Can you work these out from the drawing? Everything is in mm from the part's minimum corner. A direction names the side the tool comes from. Round coordinates to 2 decimals unless told otherwise and drop trailing zeros. Write each loop counter-clockwise with the first axis right and the second up, starting at its lowest first coordinate (ties: lowest second). Pieces come first, ordered by that corner, then holes. Notation, with made-up numbers: (-15, 13) -> (26, 13) arc R16 cw to (26, 31) -> close; hole circle Ø11 at (54, 71). An arc over 180 degrees is marked (long way). Answer as CSV lines item,"result". Start each with the question number.
Q1. For the marked faces 5, 6 and 7, which set-ups out of +Z, -Z, +X, -X, +Y, -Y let a thin tool reach every point of the face, with its end or its side?
Q2. If we mould it in two halves opening along X, with no side actions, what happens to the marked faces 1, 2, 3 and 4? For each: pulls with the +X half, pulls with the -X half, needs draft (parallel to the pull), parting line crosses it, or undercut.
Q3. If I drill on line 1 (Z direction, x = 12.7, y = 6.75); line 2 (Y direction, x = 76.5, z = 31) (1 decimal); line 3 (Y direction, x = 115.5, z = 10.5), over which ranges is the centre line in solid material (lowest first)? Write a range as [from, to].
Q4. Will these pins go through, and if not, where does the flat tip stop? pin 1 Ø17.5 at (x, z) = (9, 24.5) entering from +Y; pin 2 Ø4.5 at (x, z) = (12.7, 12.7) entering from -Y; pin 3 Ø1.6 at (y, z) = (14.5, 31.5) entering from -X (3 decimals); pin 4 Ø15 at (x, z) = (50.5, 45) entering from -Y (3 decimals).
Q5. Imagine slicing it at D-D on x = 97.5. Please give me the cut outline in (y, z).
Q6. Imagine slicing it at A-A on y = 1.75. Give the number of separate pieces and of enclosed holes in the cut face, and give its area (3 significant figures).
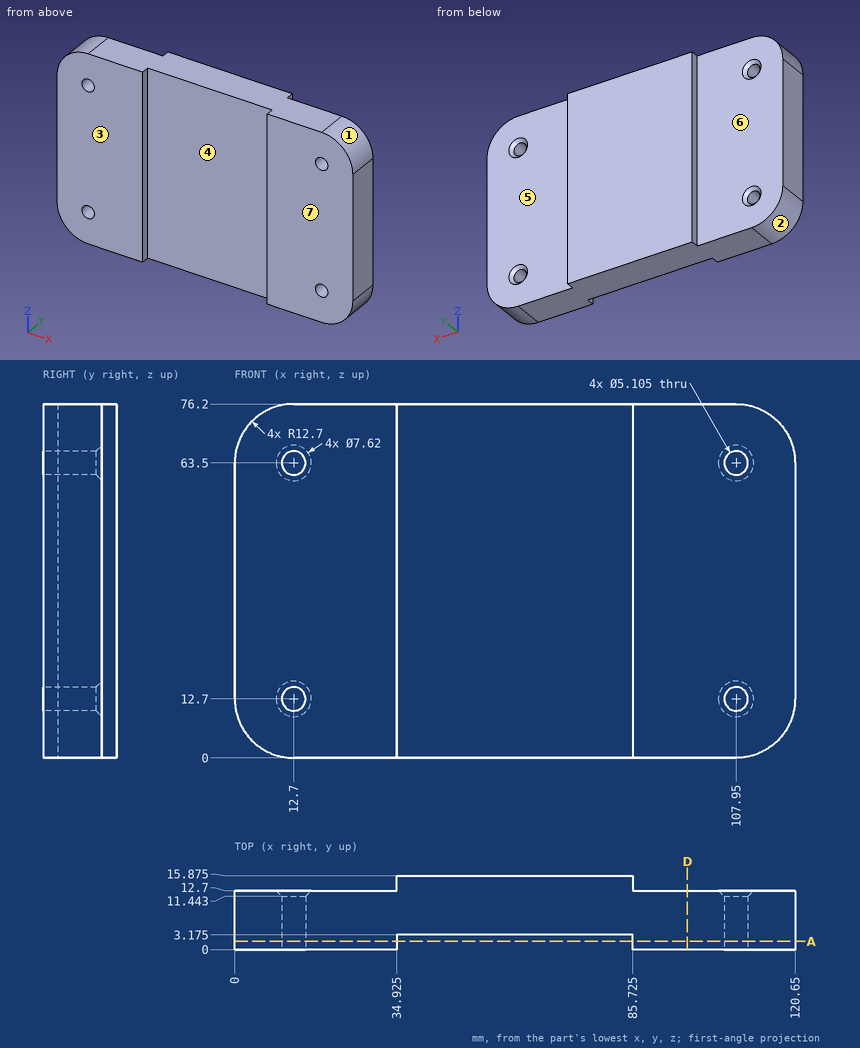
Checks:
1,face 5,"+Z, -Z, +X, +Y"
1,face 6,"+Z, -Z, -X, +Y"
1,face 7,"+Z, -Z, +X, -X, -Y"
2,face 1,"pulls with the +X half"
2,face 2,"pulls with the -X half"
2,face 3,"needs draft"
2,face 4,"undercut"
3,line 1,"[0, 10.15], [15.25, 60.95], [66.05, 76.2]"
3,line 2,"[3.2, 15.9]"
3,line 3,"[0, 12.7]"
4,pin 1,"y = 12.7"
4,pin 2,"through"
4,pin 3,"x = 34.925"
4,pin 4,"y = 3.175"
5,outline,"(0, 0) -> (12.7, 0) -> (12.7, 76.2) -> (0, 76.2) -> close"
6,separate pieces,"2"
6,enclosed holes,"4"
6,area,"5,100 mm^2"
